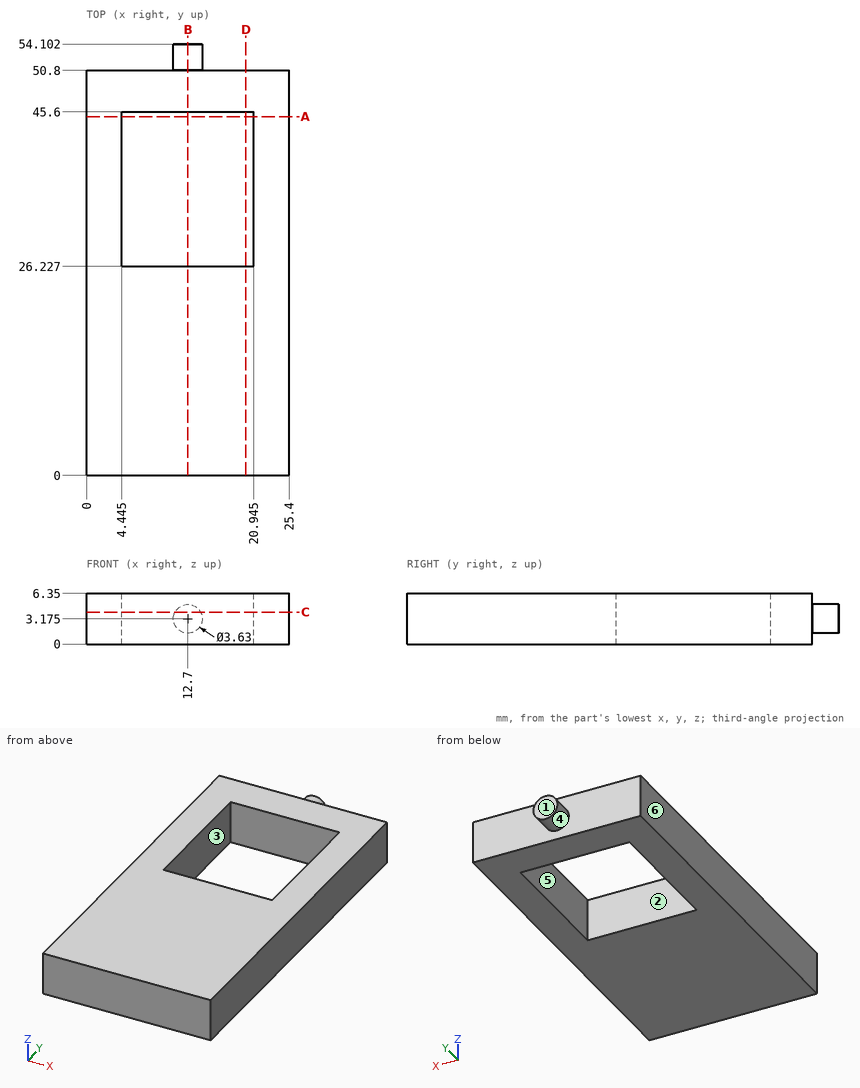
Geometry: see drawing. Coordinates: mm, zero at the bounding-box minimum. A direction names the side the tool comes from. Give positions to 0.01 mm unless a question says otherwise; leave off trailing zeros. Order: outer loops, then holes, each group sorted by start corner. A loop starts at its lowest first (then second) coordinate and runs counter-clockwise, first axis right, second up.
1. Set-up query: the marked faces 5 and 6. Return all of +Z, -Z, +X, -X, +Y, -Y with unobstructed straight access to the full face (end or side cutting, diameter ignored); none if empty.
Computed:
face 5: +Z, -Z
face 6: +Z, -Z, -X, +Y, -Y
2. Cut plane B-B (x = 12.7). Return loops of the section in (y, z).
Computed:
outline: (0, 0) - (26.23, 0) - (26.23, 6.35) - (0, 6.35) - close; (45.6, 0) - (50.8, 0) - (50.8, 1.36) - (54.1, 1.36) - (54.1, 4.99) - (50.8, 4.99) - (50.8, 6.35) - (45.6, 6.35) - close
3. Cut plane A-A (y = 45). Return loops of the section in (x, z) (3 decimals).
Computed:
outline: (0, 0) - (4.445, 0) - (4.445, 6.35) - (0, 6.35) - close; (20.945, 0) - (25.4, 0) - (25.4, 6.35) - (20.945, 6.35) - close
4. Cut plane D-D (x = 20). Return loops of the section in (y, z).
Computed:
outline: (0, 0) - (26.23, 0) - (26.23, 6.35) - (0, 6.35) - close; (45.6, 0) - (50.8, 0) - (50.8, 6.35) - (45.6, 6.35) - close
5. Line query: probe 1 along X at (y, z) = (40, 3.25) (3 decimals); probe 2 along Y at (x, z) = (17.25, 5.75); probe 3 along Y at (x, z) = (13, 3.5). Output: solid intervals per line, ascending.
Computed:
probe 1: x = 0 to 4.445, 20.945 to 25.4
probe 2: y = 0 to 26.23, 45.6 to 50.8
probe 3: y = 0 to 26.23, 45.6 to 54.1
6. Cut plane C-C (z = 4). Return loops of the section in (x, y) (1 decimal), and give its area (3 significant figures).
Computed:
outline: (0, 0) - (25.4, 0) - (25.4, 50.8) - (14.3, 50.8) - (14.3, 54.1) - (11.1, 54.1) - (11.1, 50.8) - (0, 50.8) - close; hole (4.4, 26.2) - (20.9, 26.2) - (20.9, 45.6) - (4.4, 45.6) - close
area: 981 mm2
7. Draft query along X for the marked faces 1, 2, 3 and 4. Return one class per face: released by +X, released by -X, zero draft, split by the parting line, or undercut.
Computed:
face 1: zero draft
face 2: undercut
face 3: undercut
face 4: split by the parting line
8. Pin query (flat end, axial travel): pin 1 Ø1.9 at (x, z) = (7.5, 3) entering from +Y; pin 2 Ø6 at (x, y) = (7.5, 31) entering from +Z. Return the tip coordinate at first contact, or that it passes through.
Computed:
pin 1: stops at y = 50.8
pin 2: passes through
